Geometry: final body of the model. Coordinates: model frame, mm. A direction names the side the tool comes from. Give positions to 0.01 mm unless a question says otherwise; leave off trailing zeros. Order: outer loops, then holes, each group sorted by start corner. A loop starts at its lowest first (then second) coordinate and runs counter-clockwise, first axis right, second up. Notation, with made-up numbers: M 53,-2.75 L 77,-2.75 A21 ccw 77,3.25 Z; hole C 46,87.5 d11. An arc over 180 degrees is marked long. Write item = value, one per line. Start each with the question number.
from build123d import *

# Parameters (mm, degrees)
SALIENTE_EXTRUIR1_DEPTH = 7.5
SALIENTE_EXTRUIR2_DEPTH = 15
CROQUIS7_R              = 2.5
CORTAR_EXTRUIR4_DEPTH   = 10.5
CORTAR_EXTRUIR5_START   = -3
CORTAR_EXTRUIR5_DEPTH   = 10
CHAFL_N4_SIZE           = 4
CHAFL_N5_SIZE           = 0.8


with BuildPart() as part:
    # Croquis1 → Saliente-Extruir1 (new body, symmetric)
    with BuildSketch(Plane.XY):
        with BuildLine():
            Line((-8.9, 4), (-4.936786437, 7.963213563))
            ThreePointArc((-4.936786437, 7.963213563), (-4.038051049, 5.609646436), (-2.1, 4))
            Line((-2.1, 4), (0, 4))
            Line((0, 4), (0, -4))
            ThreePointArc((0, -4), (-4.823611651, -3.031815583), (-8.9, -0.277243303))
            Line((-8.9, -0.277243303), (-8.9, 4))
        make_face()
    extrude(amount=SALIENTE_EXTRUIR1_DEPTH, both=True)

    # Croquis6 → Saliente-Extruir2 (add, through all)
    with BuildSketch(Plane(origin=(0, 0, -7.5), x_dir=(-1, 0, 0), z_dir=(0, 0, -1))):
        Polygon((0, 4), (-1.5, 5.5), (-22.5, 5.5), (-22.5, -4), (0, -4), align=None)
    extrude(amount=-SALIENTE_EXTRUIR2_DEPTH)

    # Croquis7 → Cortar-Extruir4 (cut, through all)
    with BuildSketch(Plane(origin=(0, 5.5, 0), x_dir=(1, 0, 0), z_dir=(0, 1, 0))):
        with Locations((15, 0)):
            Circle(CROQUIS7_R)
    extrude(amount=-CORTAR_EXTRUIR4_DEPTH, mode=Mode.SUBTRACT)

    # Croquis8 → Cortar-Extruir5 (cut)
    with BuildSketch(Plane(origin=(0, 5.5, 0), x_dir=(1, 0, 0), z_dir=(0, 1, 0)).offset(CORTAR_EXTRUIR5_START)):
        Polygon((15, 3.983716857), (11.55, 1.991858429), (11.55, -1.991858429), (15, -3.983716857), (18.45, -1.991858429), (18.45, 1.991858429), align=None)
    extrude(amount=-CORTAR_EXTRUIR5_DEPTH, mode=Mode.SUBTRACT)

    # Chaflán4
    chafl_n4_edges = [part.edges().sort_by_distance(p)[0] for p in [
        (22.5, 0.75, 7.5),
        (22.5, 0.75, -7.5),
    ]]
    chamfer(chafl_n4_edges, length=CHAFL_N4_SIZE)

    # Chaflán5
    chafl_n5_edges = [part.edges().sort_by_distance(p)[0] for p in [
        (12.5, 5.5, 0),
        (13.275, -4, -2.987787643),
        (11.55, -4, 0),
        (13.275, -4, 2.987787643),
        (16.725, -4, 2.987787643),
        (18.45, -4, 0),
        (16.725, -4, -2.987787643),
    ]]
    chamfer(chafl_n5_edges, length=CHAFL_N5_SIZE)


solid = part.part
1) Cut plane D-D (x = 5.5). Return loops of the section in (y, z).
2) Cut plane A-A (z = 0). Return loops of the section in (x, y).
3) Access query for faces 5 (the flat face through (18.45, 0, 0)), 6 (the flat face through (-1, 4, 0)), 7 (the flat face through (22.5, 1, 0)). Directions: +Z, -Z, +X, -X, +Y, -Y. A direction counts if a zero-diameter tool reaches every point of the face in a straight line with its end or side. Return the directions, or none.
4) Draft query along Z for faces 1 (the cylindrical face through (-4.06, 5.64, 0.11)), 2 (the flat face through (18.84, -3.59, -0.03)), 3 (the flat face through (5, 1, 7.5)), 4 (the flat face through (21, 1, -5)). Return one class per face: pulls with the +Z half, pulls with the -Z half, needs draft (parallel to the pull), parting line crosses it, or undercut.
5) Cut plane C-C (y = -0.75). Return loops of the section in (x, z), plus the area to 3 significant figures.
6) Ray query, L1, parallel to X at y = 3.8, z = 0; L2, parallel to X at y = 0.75, z = -1.25; L3, parallel to X at y = 4.75, z = -1. Return the intervals inside material, ascending.
7) Pin query (flat end, axial travel): pin 1 Ø8 at (x, z) = (5.5, 1.5) entering from +Y; pin 2 Ø1.5 at (x, y) = (1, 6.5) entering from +Z; pin 3 Ø0.6 at (x, z) = (-1, 3.5) entering from +Y; pin 4 Ø6 at (x, z) = (15, 0) entering from +Y. Return the tip coordinate at first contact, or that it passes through.
8) Cut plane B-B (z = -6). Return loops of the section in (x, y).
Reply:
q1.outline = M -4,-7.5 L 5.5,-7.5 L 5.5,7.5 L -4,7.5 Z
q2.outline = M -8.9,-0.28 A12.5 ccw 0,-4 L 10.75,-4 L 11.55,-3.2 L 11.55,2.5 L 12.5,2.5 L 12.5,4.7 L 11.7,5.5 L 1.5,5.5 L 0,4 L -2.1,4 A4.97 cw -4.94,7.96 L -8.9,4 Z; M 17.5,2.5 L 18.45,2.5 L 18.45,-3.2 L 19.25,-4 L 22.5,-4 L 22.5,5.5 L 18.3,5.5 L 17.5,4.7 Z
q3.face_5 = -Y
q3.face_6 = +Z, -Z, +Y
q3.face_7 = +Z, -Z, +X, +Y, -Y
q4.face_1 = needs draft
q4.face_2 = undercut
q4.face_3 = pulls with the +Z half
q4.face_4 = pulls with the -Z half
q5.outline = M -8.41,-7.5 L 18.5,-7.5 L 22.5,-3.5 L 22.5,3.5 L 18.5,7.5 L -8.41,7.5 Z; hole M 11.55,-1.99 L 15,-3.98 L 18.45,-1.99 L 18.45,1.99 L 15,3.98 L 11.55,1.99 Z
q5.area = 406 mm²
q6.L1 = -8.9 to 12.5, 17.5 to 22.5
q6.L2 = -8.9 to 11.55, 18.45 to 22.5
q6.L3 = -8.15 to -3.26, 0.75 to 12.65, 17.35 to 22.5
q7.pin_1 = 5.5
q7.pin_2 = through
q7.pin_3 = 4
q7.pin_4 = 5.2
q8.outline = M -8.9,-0.28 A12.5 ccw 0,-4 L 20,-4 L 20,5.5 L 1.5,5.5 L 0,4 L -2.1,4 A4.97 cw -4.94,7.96 L -8.9,4 Z
